Read the model definition and answer for the solid it produces. Units are mm, in the model's axes. A direction names the side the tool comes from. Round coordinates to 2 decimals unless told otherwise and drop trailing zeros. Order: outer loops, then holes, each group sorted by start corner. A loop starts at its lowest first (then second) coordinate and runs counter-clockwise, first axis right, second up. Notation, with made-up numbers: M 55,70 L 93,70 A23 ccw 93,103 Z; hole C 84,59.5 d11. An arc over 180 degrees is marked long. Use one line per item in the form item = value. Start each with the question number.
Autodesk Inventor part; units mm, degrees
ref_plane "YZ Plane" through (0, 0, 0) normal (1, 0, 0) x (0, 1, 0)
ref_plane "XZ Plane" through (0, 0, 0) normal (0, 1, 0) x (-1, 0, 0)
ref_plane "XY Plane" through (0, 0, 0) normal (0, 0, 1) x (1, 0, 0)
sketch "Sketch1" plane through (0, 0, 0) normal (0, 1, 0) x (-1, 0, 0)
  line L0 (-53.34, 41) -> (53.34, 41)
  line L1 (53.34, 41) -> (53.34, -41)
  line L2 (53.34, -41) -> (-53.34, -41)
  line L3 (-53.34, -41) -> (-53.34, 41)
  line L4 (-53.34, 41) -> (53.34, -41) construction
  line L5 (53.34, 41) -> (-53.34, -41) construction
  line L6 (-50.8, 32.385) -> (50.8, 32.385)
  line L7 (50.8, 32.385) -> (50.8, -32.385)
  line L8 (50.8, -32.385) -> (-50.8, -32.385)
  line L9 (-50.8, -32.385) -> (-50.8, 32.385)
  line L10 (-50.8, 32.385) -> (50.8, -32.385) construction
  line L11 (50.8, 32.385) -> (-50.8, -32.385) construction
  point P0 (0, 0)
  dimension "d0" = 106.68
  dimension "d1" = 82
  dimension "d2" = 101.6
  dimension "d3" = 64.77
extrude "Extrusion1" add sketch "Sketch1" along normal blind 5.08
sketch "Sketch2" plane through (0, 0, 0) normal (0, -1, 0) x (1, 0, 0)
  line L0 (-53.34, 41) -> (53.34, 41)
  line L1 (53.34, -41) -> (-53.34, -41)
  line L2 (53.34, 41) -> (50.7573, 41)
  line L3 (50.7573, 41) -> (50.7573, -41)
  line L4 (50.7573, -41) -> (53.34, -41)
  line L5 (53.34, -41) -> (53.34, 41)
  line L6 (-53.34, -41) -> (-50.8, -41)
  line L7 (-50.8, -41) -> (-50.8, 41)
  line L8 (-50.8, 41) -> (-53.34, 41)
  line L9 (-53.34, 41) -> (-53.34, -41)
  point P0 (0, 0)
extrude "Extrusion2" add sketch "Sketch2" along normal blind 7.62 contours L0 L7 L1 L9 | L0 L5 L1 L3
sketch "Sketch3" plane through (0, 5.08, 0) normal (0, 1, 0) x (1, 0, 0)
  line L0 (-36, -36) -> (36, -36)
  line L1 (36, -36) -> (36, 36)
  line L2 (36, 36) -> (-36, 36)
  line L3 (-36, 36) -> (-36, -36)
  line L4 (-36, -36) -> (36, 36) construction
  line L5 (36, -36) -> (-36, 36) construction
  line L6 (-36, 36) -> (-32.19, 36)
  line L7 (36, 36) -> (32.19, 36)
  line L8 (36, -36) -> (36, -40.19)
  line L9 (53.34, 41) -> (-53.34, 41)
  line L10 (-36, 41) -> (-36, 32.385)
  line L11 (50.7573, 32.385) -> (-50.8, 32.385)
  point P0 (0, 0)
  dimension "d8" = 72
  dimension "d9" = 72
sketch "Sketch4" plane through (53.34, 5.08, 41) normal (1, 0, 0) x (0, 0, -1)
  line L0 (8.615, -5.08) -> (0, -5.08)
  line L1 (0, -12.7) -> (0, 0)
  line L2 (0, -5.08) -> (0, -12.7)
  line L3 (0, -12.7) -> (0, -8.89)
  line L4 (0, -8.89) -> (82, -8.89)
  point P0 (41, -5.08)
  point P1 (82, -5.08)
  point P2 (82, -12.7)
  point P3 (41, -8.89)
hole "Hole2" at (53.34, -3.81, 0) direction (-1, 0, 0) diameter 3.81 end through all
hole "Hole3" at (-36, 5.08, 36) at (-36, 5.08, -36) at (36, 5.08, -36) at (36, 5.08, 36) direction (0, -1, 0) diameter 3.81 end through all
properties part number "Fan-Holder-4355"
Item 1: Section A-A (z = 27.5) is taken. Write down the section's boundary in (x, y), and give its area (3 significant figures).
Item 2: Section C-C (x = -19) is taken. Write down the section's boundary in (y, z) (3 decimals).
Item 3: Given P1, Ø2.5, axis at x = 36, z = -36, coming from the +Y side; P2, Ø4.5, axis at x = 36, z = 36, coming from the -Y side, each flat-ended and moving along its own axis, determine where each tip first touches the part or whether it passes through.
Item 4: Section D-D (z = 36) is taken. Write down the section's boundary in (x, y) (3 decimals).
Item 5: Section B-B (y = -3.81) is taken. Write down the section's boundary in (x, z) (3 decimals).
Item 6: For a pull along Z with two mould halves and no side action, classify faces 4 (the flat face through (1, 1, 41)), 5 (the flat face through (-50.8, -1, -1)), 6 (the flat face through (-53.34, -1, 1)), 7 (the cylindrical face through (-36.084, 2.504, 34.097)) as pulls with the +Z half, pulls with the -Z half, needs draft (parallel to the pull), parting line crosses it, or undercut.
Item 7: Find the intervals of material crossed by L1, parallel to Z at x = 36, y = 2.4 (3 decimals); L2, parallel to X at y = -5.5, z = 22; L3, parallel to Y at x = 52, z = 0 (3 decimals), in increasing order. Write a range as [from, to].
Item 8: A tool of negligible diameter and unlimited length cuts with its end or side. For faces 1 (the flat face through (50.757, -1, 1)), 2 (the flat face through (-1, 3, -32.385)), 3 (the flat face through (0, 5.08, 34)), from which of +Z, -Z, +X, -X, +Y, -Y can it reach the whole face along a straight path? Write none if from no direction.
The answers:
q1.outline = M -53.34,-7.62 L -50.8,-7.62 L -50.8,5.08 L -53.34,5.08 Z; M 50.76,-7.62 L 53.34,-7.62 L 53.34,5.08 L 50.8,5.08 L 50.8,0 L 50.76,0 Z
q1.area = 64.8 mm²
q2.outline = M 0,-41 L 5.08,-41 L 5.08,-32.385 L 0,-32.385 Z; M 0,32.385 L 5.08,32.385 L 5.08,41 L 0,41 Z
q3.P1 = through
q3.P2 = 0
q4.outline = M -53.34,-7.62 L -50.8,-7.62 L -50.8,0 L -37.905,0 L -37.905,5.08 L -53.34,5.08 Z; M -34.095,0 L 34.095,0 L 34.095,5.08 L -34.095,5.08 Z; M 37.905,0 L 50.757,0 L 50.757,-7.62 L 53.34,-7.62 L 53.34,5.08 L 37.905,5.08 Z
q5.outline = M -53.34,-41 L -50.8,-41 L -50.8,-1.905 L -53.34,-1.905 Z; M -53.34,1.905 L -50.8,1.905 L -50.8,41 L -53.34,41 Z; M 50.757,-41 L 53.34,-41 L 53.34,-1.905 L 50.757,-1.905 Z; M 50.757,1.905 L 53.34,1.905 L 53.34,41 L 50.757,41 Z
q6.face_4 = pulls with the +Z half
q6.face_5 = undercut
q6.face_6 = needs draft
q6.face_7 = undercut
q7.L1 = [-41, -37.905], [-34.095, -32.385], [32.385, 34.095], [37.905, 41]
q7.L2 = [-53.34, -50.8], [50.76, 53.34]
q7.L3 = [-7.62, -5.715], [-1.905, 5.08]
q8.face_1 = +Z, -Z, -Y
q8.face_2 = +Y, -Y
q8.face_3 = +Z, -Z, +X, -X, +Y
